```python
from build123d import *

# Parameters (mm, degrees)
SKETCH4_R           = 1.6
BOSS_EXTRUDE2_DEPTH = 1
BOSS_EXTRUDE3_DEPTH = 2.2
SKETCH6_R           = 4
SKETCH6_W           = 10.008556046
SKETCH6_H           = 9.470821567
CUT_EXTRUDE1_DEPTH  = 4.2
CUT_EXTRUDE2_DEPTH  = 10.008556
SKETCH8_W           = 2.5
SKETCH8_H           = 24.6
BOSS_EXTRUDE4_DEPTH = 10
CUT_EXTRUDE3_REACH  = 84.598
SKETCH10_R          = 4.25
CUT_EXTRUDE4_DEPTH  = 1


with BuildPart() as part:
    # Sketch4 → Boss-Extrude2 (new body)
    with BuildSketch(Plane.XY):
        Polygon((-50.042780229, 25), (8.006844837, 25), (8.006844837, 10.737807635), (28.52438473, 10.737807635), (28.52438473, 3.982032304), (32.555371359, 3.982032304), (32.555371359, -3.982032304), (28.52438473, -3.982032304), (28.52438473, -10.737807635), (8.006844837, -10.737807635), (8.006844837, -25), (-50.042780229, -25), align=None)
        with Locations((-47.542780229, 19)):
            Circle(SKETCH4_R, mode=Mode.SUBTRACT)
        with Locations((-47.542780229, -19)):
            Circle(SKETCH4_R, mode=Mode.SUBTRACT)
        with Locations((29.123529126, 0)):
            Circle(SKETCH4_R, mode=Mode.SUBTRACT)
    extrude(amount=BOSS_EXTRUDE2_DEPTH)

    # Sketch5 → Boss-Extrude3 (add)
    with BuildSketch(Plane(origin=(0, 0, 0), x_dir=(-1, 0, 0), z_dir=(0, 0, -1))):
        Polygon((10.130686795, 7.8), (-27.3, 7.8), (-27.3, -7.8), (10.130686795, -7.8), (10.416393564, -7.8), (10.416393564, -8), (10.416393564, -25), (27.916393564, -25), (27.916393564, -22.8), (42.575341492, -22.8), (42.575341492, -12.3), (50.042780229, -12.3), (50.042780229, 12.3), (42.575341492, 12.3), (42.575341492, 22.8), (10.416393564, 22.8), (10.416393564, 8), (10.416393564, 7.8), align=None)
    extrude(amount=BOSS_EXTRUDE3_DEPTH)

    # Sketch6 → Cut-Extrude1 (cut, through all)
    with BuildSketch(Plane.XY.offset(1)):
        Circle(SKETCH6_R)
        with Locations((0, -12.74225562)):
            Rectangle(SKETCH6_W, SKETCH6_H)
        with Locations((0, 12.74225562)):
            Rectangle(SKETCH6_W, SKETCH6_H)
    extrude(amount=-CUT_EXTRUDE1_DEPTH, mode=Mode.SUBTRACT)

    # Sketch7 → Cut-Extrude2 (cut)
    with BuildSketch(Plane(origin=(-5.004278023, 0, 0), x_dir=(0, 0, -1), z_dir=(1, 0, 0))):
        Polygon((0.904413332, -8.006844837), (-1, -4.814198104), (-1, -8.006844837), (0, -8.006844837), align=None)
    cut_extrude2 = extrude(amount=CUT_EXTRUDE2_DEPTH, mode=Mode.SUBTRACT)

    # Mirror1: Cut-Extrude2 across plane
    add(cut_extrude2.mirror(Plane.ZX), mode=Mode.SUBTRACT)

    # Sketch8 → Boss-Extrude4 (add)
    with BuildSketch(Plane(origin=(0, 0, -2.2), x_dir=(-1, 0, 0), z_dir=(0, 0, -1))):
        with Locations((48.792780229, 0)):
            Rectangle(SKETCH8_W, SKETCH8_H)
    extrude(amount=BOSS_EXTRUDE4_DEPTH)

    # Sketch9 → Cut-Extrude3 (cut, up to next)
    with BuildSketch(Plane.ZY.offset(50.042780229), mode=Mode.PRIVATE) as cut_extrude3_sk1:
        with BuildLine():
            Line((-9.2, 9.061272662), (-12.2, 9.061272662))
            Line((-12.2, 9.061272662), (-12.2, 5.087082771))
            Line((-12.2, 5.087082771), (-9.2, 5.087082771))
            ThreePointArc((-9.2, 5.087082771), (-7.212905055, 7.074177716), (-9.2, 9.061272662))
        make_face()
    cut_extrude3_tool1 = extrude(cut_extrude3_sk1.sketch, amount=-CUT_EXTRUDE3_REACH, mode=Mode.PRIVATE) & part.part
    add(cut_extrude3_tool1.solids().sort_by_distance((-50.04278, 7.074178, -9.898105))[0], mode=Mode.SUBTRACT)

    # Sketch10 → Cut-Extrude4 (cut)
    with BuildSketch(Plane.XY.offset(1)):
        Circle(SKETCH10_R)
    extrude(amount=-CUT_EXTRUDE4_DEPTH, mode=Mode.SUBTRACT)


solid = part.part
```
Source: CAD feature listing. Evaluate the final solid. Frame: model axes, mm. A direction names the side the tool comes from. Coordinates: 2 decimals unless noted, no trailing zeros. Loops run counter-clockwise (first coordinate to the right, second up) from the corner with the lowest first, then second, coordinate; pieces in that order, holes last. Notation, with made-up numbers: (32.5, 29.5) -> (84.5, 29.5) arc R32 cw to (84.5, 67.5) -> close; hole circle Ø2 at (-33.75, 85). An arc over 180 degrees is marked (long way). One line per item, written item: value. Start each with the question number.
Q1. Contact query for flat-ended pins moving along their axis: P1, Ø5, axis at x = -47.54, y = -19, coming from the -Z side; P2, Ø1, axis at x = -40, y = 19.5, coming from the -Z side; P3, Ø0.8, axis at x = 31.5, z = 0.5, coming from the +Y side. Output: stop coordinate, or through.
Q2. Section query A-A, the plane y = 0. Return the cut outline in (x, z), and give its area (3 significant figures).
Q3. Line query: line 1 along Y through (x, z) = (0, -0.9); line 2 along Z through (x, y) = (-11, 2); line 3 along Y through (x, z) = (0, 0.7). Output: solid intervals per line, ascending.
Q4. Section query C-C, the plane z = -10.75. Return the cut outline in (x, y).
Q5. Section query D-D, the plane y = -19. Return the cut outline in (x, z).
Q6. Mould query, pull axis Y, two halves, no side actions, for faces 5 (the face through (-49, 5.087, -11)), 6 (the face through (-35, -22.8, -1)), 7 (the face through (8, 7.8, -1)). Classes: pulls with the +Y half, pulls with the -Y half, needs draft (parallel to the pull), parting line crosses it, or undercut.
Q7. Section query B-B, the plane x = 0. Return the cut outline in (y, z), and give its area (3 significant figures).
Q8. Set-up query: faces 1 (the face through (27.3, 0, -1)), 2 (the face through (9, -7.8, -1)), 3 (the face through (-42.575, -18, -1)), 4 (the face through (-0.07, -6.328, 0.097)). Return all of +Z, -Z, +X, -X, +Y, -Y with unobstructed straight access to the full face (end or side cutting, diameter ignored); none if empty.
Results:
1. P1: z = 0
1. P2: z = -2.2
1. P3: y = 3.98
2. outline: (-50.04, -12.2) -> (-47.54, -12.2) -> (-47.54, -2.2) -> (-4, -2.2) -> (-4, 0) -> (-4.25, 0) -> (-4.25, 1) -> (-50.04, 1) -> close; (4, -2.2) -> (27.3, -2.2) -> (27.3, 0) -> (27.52, 0) -> (27.52, 1) -> (4.25, 1) -> (4.25, 0) -> (4, 0) -> close; (30.72, 0) -> (32.56, 0) -> (32.56, 1) -> (30.72, 1) -> close
2. area: 248 mm^2
3. line 1: -7.8 to -4, 4 to 7.8
3. line 2: -2.2 to 1
3. line 3: -25 to -17.48, -5.32 to -4.25, 4.25 to 5.32, 17.48 to 25
4. outline: (-50.04, -12.3) -> (-47.54, -12.3) -> (-47.54, 5.09) -> (-50.04, 5.09) -> close; (-50.04, 9.06) -> (-47.54, 9.06) -> (-47.54, 12.3) -> (-50.04, 12.3) -> close
5. outline: (-50.04, 0) -> (-49.14, 0) -> (-49.14, 1) -> (-50.04, 1) -> close; (-45.94, 0) -> (-42.58, 0) -> (-42.58, -2.2) -> (-10.42, -2.2) -> (-10.42, 0) -> (8.01, 0) -> (8.01, 1) -> (-45.94, 1) -> close
6. face 5: undercut
6. face 6: pulls with the -Y half
6. face 7: pulls with the +Y half
7. outline: (-25, 0) -> (-17.48, 0) -> (-17.48, 1) -> (-25, 1) -> close; (-7.8, -2.2) -> (-4, -2.2) -> (-4, 0) -> (-4.25, 0) -> (-4.25, 1) -> (-4.81, 1) -> (-7.8, -0.78) -> close; (4, -2.2) -> (7.8, -2.2) -> (7.8, -0.78) -> (4.81, 1) -> (4.25, 1) -> (4.25, 0) -> (4, 0) -> close; (17.48, 0) -> (25, 0) -> (25, 1) -> (17.48, 1) -> close
7. area: 33.5 mm^2
8. face 1: -Z, +X, +Y, -Y
8. face 2: -Z, +X, -Y
8. face 3: -Z, -X, -Y
8. face 4: +Z
